Design review of the part shown in the three views and the two pictorial views. Dimensions are in mm from the part's minimum x, y and z. A direction names the side the tool comes from. Round coordinates to 2 decimals unless told otherwise and drop trailing zeros. Loops run counter-clockwise (first coordinate to the right, second up) from the corner with the lowest first, then second, coordinate; pieces in that order, holes last. Notation, with made-up numbers: (38.25, -17) - (43.25, -17) arc R33 ccw to (43.25, 12) - close; hole circle Ø3 at (21, -10.75). An arc over 180 degrees is marked (long way). Return JSON: item names as keys, results as strings. Group by question number.
(1) For the marked faces 4, 5, 6, 7 and 8, list the 3-axis set-ups (+Z, -Z, +X, -X, +Y, -Y) from which the entire face can be reached by the end or side of a thin tool; tool diameter is ignored.
(2) We need section A-A, the plane x = 11.5. Write out the cut boundary in (y, z).
(3) Wall thickness on L1, parallel to X at y = 3.4, z = 19; L2, parallel to Y at x = 15.5, z = 15.5; L3, parallel to X at y = 12.75, z = 7: over which ranges is each line inside the solid? List them lowest first. Write a range as [from, to].
(4) The part is to be moulded in two halves that separate along X. For the marked faces 1, 2 and 3, say which applies: pulls with the +X half, pulls with the -X half, needs draft (parallel to the pull), parting line crosses it, or undercut.
(5) We need section D-D, the plane y = 1.5. Write out the cut boundary in (x, z).
(6) Clearance check with flat-ended pins moving along their axes: pin 1 (12 mm diameter, centred on x = 6, z = 7, fed in from -Y); pin 2 (5 mm diameter, centred on x = 4.5, y = 7.5, fed in from +Z); pin 3 (4 mm diameter, centred on x = 11.5, z = 17, fed in from +Y); pin 4 (3.5 mm diameter, centred on y = 7, z = 10, fed in from +X). State where each tip first meets the part, or that it passes through.
(7) We need section B-B, the plane x = 16. Write out the cut boundary in (y, z), and give its area (3 significant figures).
(8) We need section C-C, the plane z = 16. Write out the cut boundary in (x, y), and give its area (3 significant figures).
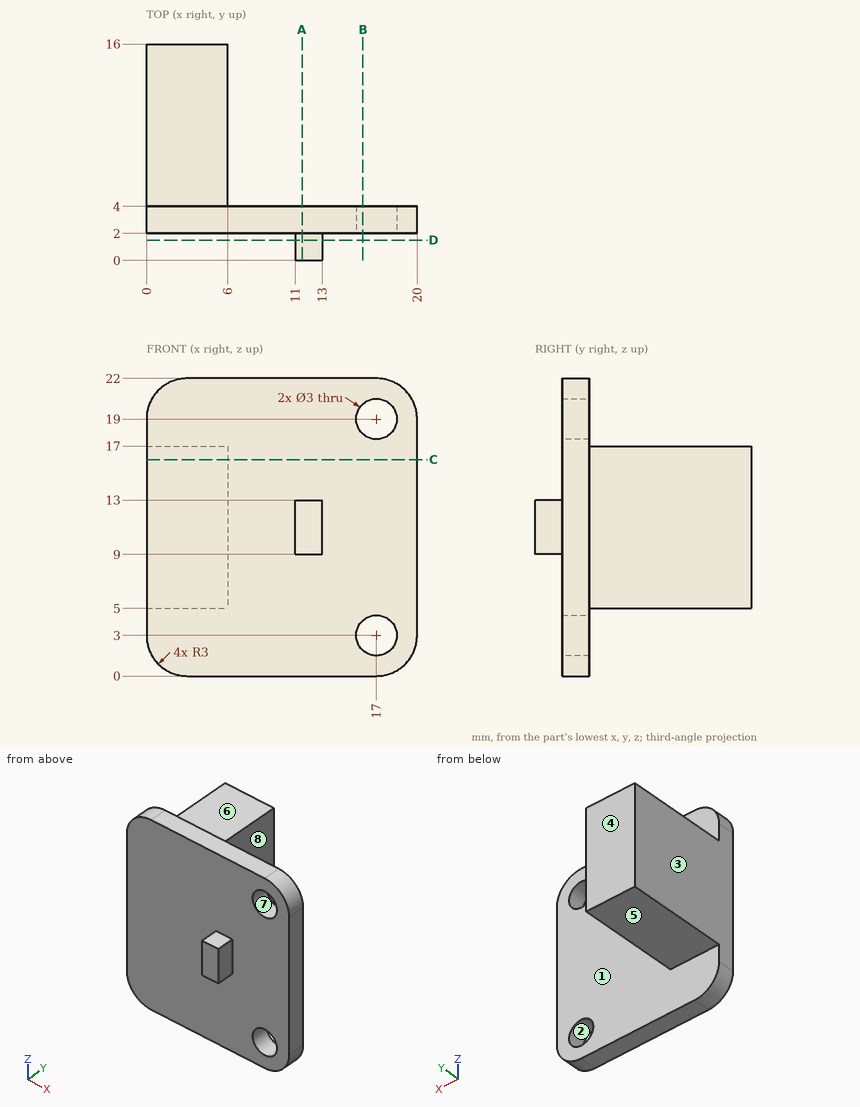
Solutions:
{
 "1": {"face 4": "+Z, -Z, +X, -X, +Y", "face 5": "-Z, +X, -X, +Y", "face 6": "+Z, +X, -X, +Y", "face 7": "+Y, -Y", "face 8": "+Z, -Z, +X, +Y"},
 "2": {"outline": "(0, 9) - (2, 9) - (2, 0) - (4, 0) - (4, 22) - (2, 22) - (2, 13) - (0, 13) - close"},
 "3": {"L1": "[0, 15.5], [18.5, 20]", "L2": "[2, 4]", "L3": "[0, 6]"},
 "4": {"face 1": "needs draft", "face 2": "undercut", "face 3": "pulls with the -X half"},
 "5": {"outline": "(11, 9) - (13, 9) - (13, 13) - (11, 13) - close"},
 "6": {"pin 1": "y = 0", "pin 2": "z = 17", "pin 3": "y = 4", "pin 4": "x = 6"},
 "7": {"outline": "(2, 0) - (4, 0) - (4, 1.88) - (2, 1.88) - close; (2, 4.12) - (4, 4.12) - (4, 17.88) - (2, 17.88) - close; (2, 20.12) - (4, 20.12) - (4, 22) - (2, 22) - close", "area": "35.1 mm^2"},
 "8": {"outline": "(0, 2) - (20, 2) - (20, 4) - (6, 4) - (6, 16) - (0, 16) - close", "area": "112 mm^2"}
}
